from build123d import *

# Parameters (mm, degrees)
BOSS_EXTRU_1_DEPTH      = 20
ESQUISSE1_R             = 1
ENL_V_MAT_EXTRU_1_DEPTH = 6.695841166
BOSS_EXTRU_2_DEPTH      = 20
ESQUISSE3_R             = 1.25
ENL_V_MAT_EXTRU_2_DEPTH = 21


with BuildPart() as part:
    # ProfileRainureEsquisse → Boss.-Extru.1 (new body)
    with BuildSketch(Plane.XY):
        Polygon((0, 0), (0, 5), (4, 8), (4, 5), (5.695841166, 5), (5.695841166, 0), (4, 0), (4, -3), align=None)
    extrude(amount=BOSS_EXTRU_1_DEPTH)

    # Esquisse1 → Enlèv. mat.-Extru.1 (cut, through all)
    with BuildSketch(Plane(origin=(5.695841166, 0, 0), x_dir=(0, 0, -1), z_dir=(1, 0, 0))):
        with Locations((-10, 2.5)):
            Circle(ESQUISSE1_R)
    extrude(amount=-ENL_V_MAT_EXTRU_1_DEPTH, mode=Mode.SUBTRACT)

    # Esquisse2 → Boss.-Extru.2 (add)
    with BuildSketch(Plane(origin=(5.695841166, 0, 0), x_dir=(0, 0, -1), z_dir=(1, 0, 0))):
        Polygon((-14, 0), (-14, 5), (-17.8, 8), (-17.8, 5), (-20, 5), (-20, 0), (-17.8, 0), (-17.8, -3), align=None)
        Polygon((-6, 5), (-6, 0), (-2.2, -3), (-2.2, 0), (0, 0), (0, 5), (-2.2, 5), (-2.2, 8), align=None)
    extrude(amount=BOSS_EXTRU_2_DEPTH)

    # Esquisse3 → Enlèv. mat.-Extru.2 (cut, through all)
    with BuildSketch(Plane.XY.offset(20)):
        with Locations((15.695841166, 2.5)):
            Circle(ESQUISSE3_R)
    extrude(amount=-ENL_V_MAT_EXTRU_2_DEPTH, mode=Mode.SUBTRACT)


solid = part.part
Input: part model. Units: mm. Frame: model coordinates. A direction names the side the tool comes from. Coordinates: 2 decimals unless noted, no trailing zeros. Order: outer loops, then holes, each group sorted by start corner. A loop starts at its lowest first (then second) coordinate and runs counter-clockwise, first axis right, second up. Notation, with made-up numbers: M 72,11.5 L 104,11.5 A26 cw 104,28.5 Z; hole C -38.5,5.5 d8. An arc over 180 degrees is marked long. Answer as CSV lines item,"result".
1. Section B-B (z = 10). Return the cut outline in (x, y), then the cut area to 3 significant figures.
Reported:
outline,"M 0,0 L 4,-3 L 4,0 L 5.7,0 L 5.7,1.5 L 0,1.5 Z; M 0,3.5 L 5.7,3.5 L 5.7,5 L 4,5 L 4,8 L 0,5 Z"
area,"29.1 mm2"
2. Material intervals for line 1 (Z direction, x = 21.5, y = 0.25); line 2 (Y direction, x = 16.5, z = 1.75); line 3 (X direction, y = 3.25, z = 12.25), sorted ascending. Write a range as from..to.
Reported:
line 1,"0..6, 14..20"
line 2,"0..1.54, 3.46..5"
line 3,"0..5.7"
3. First-contact query: P1, Ø2.5, axis at x = 15, y = 1.5, coming from the -Z side; P2, Ø0.9, axis at y = -1, z = 4.5, coming from the -X side; P3, Ø1.6, axis at y = 2.5, z = 10, coming from the +X side; P4, Ø0.9, axis at x = 13, y = 6, coming from the -Z side. Flat tips, straight axial feed; report the tip coordinate or a pass-through.
Reported:
P1,"z = 0"
P2,"x = 0.73"
P3,"through"
P4,"z = 2.2"
4. Section C-C (y = 2.5). Return the cut outline in (x, z), then the cut area to 3 significant figures.
Reported:
outline,"M 0,0 L 14.45,0 L 14.45,6 L 5.7,6 L 5.7,9 L 0,9 Z; M 0,11 L 5.7,11 L 5.7,14 L 14.45,14 L 14.45,20 L 0,20 Z; M 16.95,0 L 25.7,0 L 25.7,6 L 16.95,6 Z; M 16.95,14 L 25.7,14 L 25.7,20 L 16.95,20 Z"
area,"313 mm2"
5. Section A-A (y = 6.5). Return the cut outline in (x, z), then the cut area to 3 significant figures.
Reported:
outline,"M 2,0 L 4,0 L 4,20 L 2,20 Z; M 5.7,2.2 L 25.7,2.2 L 25.7,4.1 L 5.7,4.1 Z; M 5.7,15.9 L 25.7,15.9 L 25.7,17.8 L 5.7,17.8 Z"
area,"116 mm2"
6. Section D-D (z = 15.5). Return the cut outline in (x, y).
Reported:
outline,"M 0,0 L 4,-3 L 4,0 L 5.7,0 L 5.7,-1.18 L 25.7,-1.18 L 25.7,6.18 L 5.7,6.18 L 5.7,5 L 4,5 L 4,8 L 0,5 Z; hole C 15.7,2.5 d2.5"
7. Access query for faces 4 (the flat face through (16, 6, 2.2)), 5 (the flat face through (16, -1, 17.8)), 6 (the flat face through (4, 7, 10)). Directions: +Z, -Z, +X, -X, +Y, -Y. A direction counts if a zero-diameter tool reaches every point of the face in a straight line with its end or side. Return the directions, or none.
Reported:
face 4,"-Z, +X, +Y"
face 5,"+Z, +X, -Y"
face 6,"+Z, -Z, +Y"
8. Pull-direction query (Z, two-part tool) for faces 1 (the flat face through (15.6, -1.5, 4.1)), 2 (the flat face through (13, 3, 20)), 3 (the flat face through (5.696, -1, 3)); classes: released by +Z, released by -Z, zero draft, split by the parting line, or undercut.
Reported:
face 1,"undercut"
face 2,"released by +Z"
face 3,"zero draft"
